Work out the finished part from the listing and answer in its coordinate system (mm). Face numbers are marked on the shaded views. Give positions to 0.01 mm unless a question says otherwise; leave off trailing zeros. Loops run counter-clockwise (first coordinate to the right, second up) from the corner with the lowest first, then second, coordinate; pieces in that order, holes last.
```python
from build123d import *

# Parameters (mm, degrees)
F1_DEPTH      = 25
F3_DEPTH      = 12.501
F4_DEPTH      = 12.501
F7_DEPTH      = 270
F7_DEPTH_BACK = 45
F8_T1_DEPTH   = 45
F8_T3_DEPTH   = 5
F9_R          = 5
F10_R         = 1
F12_D         = 3


# Not quite as in the source:
# - a fillet or chamfer that OpenCascade refuses, or shapes differently, is made with other operations: its cross-section is extruded or revolved along the edge and cut away or added


with BuildPart() as f1:
    # F0 (on Front) → F1 (new body)
    with BuildSketch(Plane.XZ):
        with BuildLine():
            ThreePointArc((-35.5866095653, 3), (-41.8366095653, -3.25), (-35.5866095653, -9.5))
            Line((-35.5866095653, -9.5), (63.9133904347, -9.5))
            Line((63.9133904347, -9.5), (63.9133904347, -6.5))
            Line((63.9133904347, -6.5), (-35.5866095653, -6.5))
            ThreePointArc((-35.5866095653, -6.5), (-38.8366095653, -3.25), (-35.5866095653, 0))
            Line((-35.5866095653, 0), (-6.0866095653, 0))
            Line((-6.0866095653, 0), (-6.0866095653, 3))
            Line((-6.0866095653, 3), (-35.5866095653, 3))
        make_face()
    extrude(amount=F1_DEPTH)

    # F2 (on face) → F3 (cut, through all)
    with BuildSketch(Plane.XY.offset(3)):
        with BuildLine():
            ThreePointArc((-32.153940115, -14), (-25.3310686782, -18.7041645665), (-19.8366095653, -12.5))
            ThreePointArc((-19.8366095653, -12.5), (-25.3310686782, -6.2958354335), (-32.153940115, -11))
            ThreePointArc((-32.153940115, -11), (-32.3366095653, -12.5), (-32.153940115, -14))
        make_face()
    extrude(amount=-F3_DEPTH, mode=Mode.SUBTRACT)

    # F2 (on face) → F4 (cut, through all)
    with BuildSketch(Plane.XY.offset(3)):
        with BuildLine():
            ThreePointArc((-32.153940115, -14), (-25.3310686782, -18.7041645665), (-19.8366095653, -12.5))
            ThreePointArc((-19.8366095653, -12.5), (-25.3310686782, -6.2958354335), (-32.153940115, -11))
            ThreePointArc((-32.153940115, -11), (-32.3366095653, -12.5), (-32.153940115, -14))
        make_face()
        with BuildLine():
            ThreePointArc((-32.153940115, -14), (-32.3366095653, -12.5), (-32.153940115, -11))
            Line((-32.153940115, -11), (-41.9135839269, -11))
            Line((-41.9135839269, -11), (-41.9135839269, -14))
            Line((-41.9135839269, -14), (-32.153940115, -14))
        make_face()
    extrude(amount=-F4_DEPTH, mode=Mode.SUBTRACT)

    # F6 (on offset) → F7 (join, two sides)
    with BuildSketch(Plane.YZ.offset(58.9133904347)) as f7_sk:
        with BuildLine():
            ThreePointArc((-12.4225467883, -6.5), (-10.3514703126, -5.5947574316), (-9.5, -3.501))
            ThreePointArc((-9.5, -3.501), (-14.5937574316, -1.3524703126), (-12.5774532117, -6.5))
            Line((-12.5774532117, -6.5), (-12.4225467883, -6.5))
        make_face()
        with BuildLine():
            Line((-12.4225467883, -6.5), (-12.5774532117, -6.5))
            ThreePointArc((-12.5774532117, -6.5), (-12.5, -6.501), (-12.4225467883, -6.5))
        make_face()
    extrude(amount=F7_DEPTH)
    extrude(f7_sk.sketch, amount=-F7_DEPTH_BACK)

    # F8: fillet of radius 3 on 4 edges, made by hand

    # F8_s2 → F8_t1 (join)
    with BuildSketch(Plane.YZ.offset(13.9133904347)):
        with BuildLine():
            ThreePointArc((-18.5001459648, -6.5004), (-16.3786421293, -5.6217630236), (-15.4995999453, -3.5004270532))
            Line((-15.4995999453, -3.5004270532), (-15.1995453433, -3.500484366))
            ThreePointArc((-15.1995453433, -3.500484366), (-14.4336951193, -5.3852845615), (-12.5697064807, -6.2000454108))
            Line((-12.5697064807, -6.2000454108), (-12.5774532117, -6.8000546074))
            ThreePointArc((-12.5774532117, -6.8000546074), (-15.5387995882, -6.8000546074), (-18.5001459648, -6.8004546074))
            Line((-18.5001459648, -6.8004546074), (-18.5001459648, -6.5004))
        make_face()
        with BuildLine():
            ThreePointArc((-6.4998540352, -6.5004), (-8.6213578707, -5.6217630236), (-9.5004000547, -3.5004270532))
            Line((-9.5004000547, -3.5004270532), (-9.8004546567, -3.500484366))
            ThreePointArc((-9.8004546567, -3.500484366), (-10.5663048807, -5.3852845615), (-12.4302935193, -6.2000454108))
            Line((-12.4302935193, -6.2000454108), (-12.4225467883, -6.8000546074))
            ThreePointArc((-12.4225467883, -6.8000546074), (-9.4612004118, -6.8000546074), (-6.4998540352, -6.8004546074))
            Line((-6.4998540352, -6.8004546074), (-6.4998540352, -6.5004))
        make_face()
    extrude(amount=F8_T1_DEPTH)

    # F8_s4 → F8_t3 (join)
    with BuildSketch(Plane.YZ.offset(58.9133904347)):
        with BuildLine():
            ThreePointArc((-18.5001459648, -6.5004), (-16.3786421293, -5.6217630236), (-15.4995999453, -3.5004270532))
            Line((-15.4995999453, -3.5004270532), (-15.1995453433, -3.500484366))
            ThreePointArc((-15.1995453433, -3.500484366), (-14.4336951193, -5.3852845615), (-12.5697064807, -6.2000454108))
            Line((-12.5697064807, -6.2000454108), (-12.5774532117, -6.8000546074))
            ThreePointArc((-12.5774532117, -6.8000546074), (-15.5387995882, -6.8000546074), (-18.5001459648, -6.8004546074))
            Line((-18.5001459648, -6.8004546074), (-18.5001459648, -6.5004))
        make_face()
        with BuildLine():
            ThreePointArc((-6.4998540352, -6.5004), (-8.6213578707, -5.6217630236), (-9.5004000547, -3.5004270532))
            Line((-9.5004000547, -3.5004270532), (-9.8004546567, -3.500484366))
            ThreePointArc((-9.8004546567, -3.500484366), (-10.5663048807, -5.3852845615), (-12.4302935193, -6.2000454108))
            Line((-12.4302935193, -6.2000454108), (-12.4225467883, -6.8000546074))
            ThreePointArc((-12.4225467883, -6.8000546074), (-9.4612004118, -6.8000546074), (-6.4998540352, -6.8004546074))
            Line((-6.4998540352, -6.8004546074), (-6.4998540352, -6.5004))
        make_face()
    extrude(amount=F8_T3_DEPTH)

    # F9
    f9_edges = [f1.edges().sort_by_distance(p)[0] for p in [
        (63.91339, -25, -8),
        (63.91339, 0, -8),
        (-6.08661, 0, 1.5),
        (-6.08661, -25, 1.5),
    ]]
    fillet(f9_edges, radius=F9_R)

    # F10
    f10_edges = [f1.edges().sort_by_distance(p)[0] for p in [
        (328.91339, -15.5, -3.501),
    ]]
    fillet(f10_edges, radius=F10_R)

    # F12 (through all)
    with Locations(Plane(origin=(0, 0, 0), x_dir=(1, 0, 0), z_dir=(0, 1, 0))):
        with Locations((316.4133904347, 3.501)):
            Hole(F12_D / 2)


solid = f1.part
```
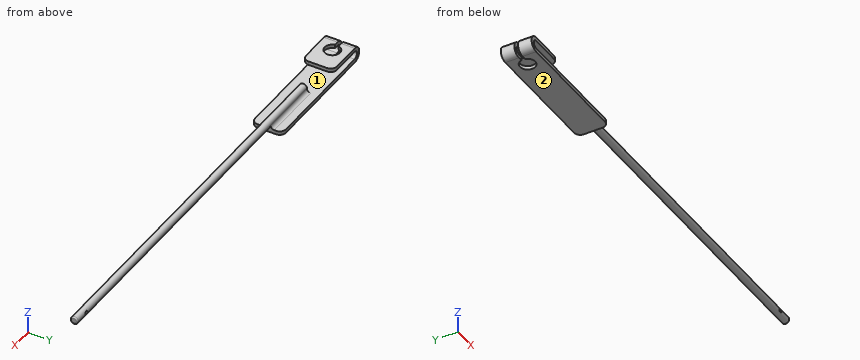
Q1. Determine the mould class of the marked faces 1 and 2 for opening direction Z: +Z half, -Z half, draft (parallel to the pull), parting line (faces both ways), or undercut.
Q2. Consider line 1 along Z through (x, y) = (-17, -8.5); line 2 along Y through (x, z) = (144.5, -4); line 3 along X through (y, z) = (-12, -4.5). Determine where each line is inside the solid, lowest interval first.
Q3. Given pin 1 (3.5 mm diameter, centred on x = 316.41, z = -3.5, fed in from +Y); pin 2 (4 mm diameter, centred on x = 290.5, y = -11, fed in from -Z); pin 3 (1 mm diameter, centred on y = -5, z = -4, fed in from +X), each flat-ended and moving along its own axis, determine where each tip first touches the part or whether it passes through.
Q4. Section A-A on x = 222.5 is taken. Give the vertices of the cut face in (y, z), plus the area to 3 significant figures.
Check result:
1. face 1: undercut
1. face 2: -Z half
2. line 1: z = -9.5 to -6.5, 0 to 3
2. line 2: y = -15.46 to -9.54
2. line 3: x = 13.91 to 315.29, 317.53 to 328.91
3. pin 1: stops at y = -9.5
3. pin 2: stops at z = -6.5
3. pin 3: stops at x = -38.59
4. outline: circle Ø6 at (-12.5, -3.5)
4. area: 28.3 mm2
